from build123d import *

# Parameters (mm, degrees)
F2_DEPTH = 12.5
F3_R     = 33.2218818367
F4_DEPTH = 39.2
F5_R     = 1


with BuildPart() as f1:
    # F0 (on Front) → F1 (revolve)
    with BuildSketch(Plane.XZ):
        Polygon((33.2218818367, 44.7680167854), (-7.1723973379, 44.7680167854), (-7.1723973379, 39.0236787498), (-7.1723973379, 0), (33.2218818367, 0), align=None)
    revolve(axis=Axis((33.2218818367, 0, 22.3840083927), (0, 0, -1)))

    # F0 (on Front) → F2 (join, symmetric)
    with BuildSketch(Plane.XZ):
        Polygon((-32.3489792645, 44.7680167854), (-32.3489792645, 0), (-22.3954468966, 0), (-22.3954468966, 39.0236787498), (-7.1723973379, 39.0236787498), (-7.1723973379, 44.7680167854), (-22.3954468966, 44.7680167854), align=None)
        Polygon((33.2218818367, 44.7680167854), (-7.1723973379, 44.7680167854), (-7.1723973379, 39.0236787498), (-7.1723973379, 0), (33.2218818367, 0), align=None)
    extrude(amount=F2_DEPTH, both=True)

    # F3 (on face) → F4 (cut)
    with BuildSketch(Plane.XY.offset(44.7680167854)):
        with Locations((33.2218818367, 0)):
            Circle(F3_R)
    extrude(amount=-F4_DEPTH, mode=Mode.SUBTRACT)

    # F5
    f5_edges = [f1.edges().sort_by_distance(p)[0] for p in [
        (73.616161, 0, 44.768017),
        (0, 0, 44.768017),
        (-18.769328, 12.5, 44.768017),
        (-32.348979, 0, 44.768017),
        (-18.769328, -12.5, 44.768017),
        (-5.189676, -12.5, 22.384008),
        (-6.181037, -12.5, 0),
        (-7.172397, -12.5, 19.511839),
        (-14.783922, -12.5, 39.023679),
        (-22.395447, -12.5, 19.511839),
        (-27.372213, -12.5, 0),
        (-32.348979, -12.5, 22.384008),
        (-32.348979, 12.5, 22.384008),
        (-32.348979, 0, 0),
        (-5.189676, 12.5, 22.384008),
        (-6.181037, 12.5, 0),
        (-7.172397, 12.5, 19.511839),
        (-14.783922, 12.5, 39.023679),
        (-22.395447, 12.5, 19.511839),
        (-27.372213, 12.5, 0),
        (73.616161, 0, 0),
        (-7.172397, 0, 0),
        (-22.395447, 0, 0),
    ]]
    fillet(f5_edges, radius=F5_R)


solid = f1.part
Read the model definition and answer for the solid it produces. Units are mm, in the model's axes. A direction names the side the tool comes from. Give positions to 0.01 mm unless a question says otherwise; leave off trailing zeros. Write each loop counter-clockwise with the first axis right and the second up, starting at its lowest first coordinate (ties: lowest second). Pieces come first, ordered by that corner, then holes. Notation, with made-up numbers: (32.5, -38) - (58.5, -38) arc R34 cw to (58.5, -7) - close; hole circle Ø8 at (49.5, 44.25). An arc over 180 degrees is marked (long way). Use CSV: the item, a comma, the result in double quotes. Start each with the question number.
(1) Given P1, Ø12.5, axis at x = -17, z = 26.5, coming from the +Y side; P2, Ø1, axis at x = -8.5, z = 22.5, coming from the -Y side; P3, Ø1.5, axis at x = 45.5, z = 32, coming from the -Y side; P4, Ø1.5, axis at x = 7.5, z = 33, coming from the +Y side, each flat-ended and moving along its own axis, determine where each tip first touches the part or whether it passes through.
(2) Determine the mould class of faces 4 (the flat face through (-27, 0, 0)), 5 (the cylindrical face through (73.585, 1.588, 22.085)), 6 (the flat face through (-32.349, 0, 23)), 7 (the flat face through (-15, 0, 39.024)) for opening direction X: +X half, -X half, draft (parallel to the pull), parting line (faces both ways), or undercut.
(3) Find section B-B (y = 0). Give the vertices of the cut face in (x, z), plus the area to 3 significant figures.
(4) Find section A-A (z = 17). Give the vertices of the cut face in (x, y), plus the area to 3 significant figures.
(5) For faces 1 (the flat face through (-24, -12.5, 27)), 2 (the flat face through (-7.172, 0, 20)), 3 (the cylindrical face through (64.91, 9.98, 24.94)), determine the directions among +Z, -Z, +X, -X, +Y, -Y from which every point of the face is accessible in a straight line to the end or side of a thin tool.
(6) Consider line 1 along X through (y, z) = (-0.5, 13); line 2 along X through (y, z) = (-6.5, 22.5); line 3 along Y through (x, z) = (6.5, 18.5). Determine where each line is inside the solid, lowest interval first.
Findings below:
1,P1,"y = 12.49"
1,P2,"through"
1,P3,"y = -38.71"
1,P4,"y = 31.75"
2,face 4,"draft"
2,face 5,"parting line"
2,face 6,"-X half"
2,face 7,"undercut"
3,outline,"(-32.35, 1) arc R1 ccw to (-31.35, 0) - (-23.4, 0) arc R1 ccw to (-22.4, 1) - (-22.4, 39.02) - (-7.17, 39.02) - (-7.17, 1) arc R1 ccw to (-6.17, 0) - (72.62, 0) arc R1 ccw to (73.62, 1) - (73.62, 43.77) arc R1 ccw to (72.62, 44.77) - (67.44, 44.77) arc R1 ccw to (66.44, 43.77) - (66.44, 5.57) - (0, 5.57) - (0, 43.77) arc R1 ccw to (-1, 44.77) - (-31.35, 44.77) arc R1 ccw to (-32.35, 43.77) - close"
3,area,"1,540 mm2"
4,outline,"(-32.35, -11.5) arc R1 ccw to (-31.35, -12.5) - (-23.4, -12.5) arc R1 ccw to (-22.4, -11.5) - (-22.4, 11.5) arc R1 ccw to (-23.4, 12.5) - (-31.35, 12.5) arc R1 ccw to (-32.35, 11.5) - close; (-7.17, -11.5) arc R1 ccw to (-6.17, -12.5) - (-5.91, -12.5) arc R1 cw to (-4.96, -13.17) arc R40.39 ccw (long way) to (-4.96, 13.17) arc R1 cw to (-5.91, 12.5) - (-6.17, 12.5) arc R1 ccw to (-7.17, 11.5) - close; hole circle Ø66.44 at (33.22, 0)"
4,area,"1,920 mm2"
5,face 1,"+Z, -Z, -X, -Y"
5,face 2,"-Z, +Y, -Y"
5,face 3,"+Z"
6,line 1,"-32.35 to -22.4, -7.17 to 0, 66.44 to 73.61"
6,line 2,"-32.35 to -22.4, -7.17 to 0.64, 65.8 to 73.09"
6,line 3,"-30.29 to -19.74, 19.74 to 30.29"
